Design review of the part built by this model. Coordinates are the model's own, in mm. Face numbers are marked on the shaded views. A direction names the side the tool comes from. Give positions to 0.01 mm unless a question says otherwise; leave off trailing zeros. Order: outer loops, then holes, each group sorted by start corner. A loop starts at its lowest first (then second) coordinate and runs counter-clockwise, first axis right, second up. Notation, with made-up numbers: (63.25, 89.25) - (97.25, 89.25) arc R21 cw to (97.25, 117.25) - close; hole circle Ø5 at (-13, 58.5). An arc over 180 degrees is marked (long way). Write each question's results on one line, items separated by ' | '. Start each with the question number.
```python
from build123d import *

# Parameters (mm, degrees)
F0_R     = 50
F0_R_2   = 15
F4_DEPTH = 30
F1_T     = -2.5
F2_W     = 3
F2_H     = 99.95499
F5_DEPTH = 27.5


with BuildPart() as f4:
    # F0 (on Top) → F4 (new body)
    with BuildSketch(Plane.XY):
        Circle(F0_R)
        Circle(F0_R_2, mode=Mode.SUBTRACT)
    extrude(amount=F4_DEPTH)

    # F1
    f1_openings = [f4.faces().sort_by_distance(p)[0] for p in [
        (-48.585786, 0, 30),
    ]]
    offset(amount=F1_T, openings=f1_openings)

    # F2 (on face) → F5 (join)
    with BuildSketch(Plane.XY.offset(2.5)):
        Rectangle(F2_W, F2_H)
    extrude(amount=F5_DEPTH)


solid = f4.part
```
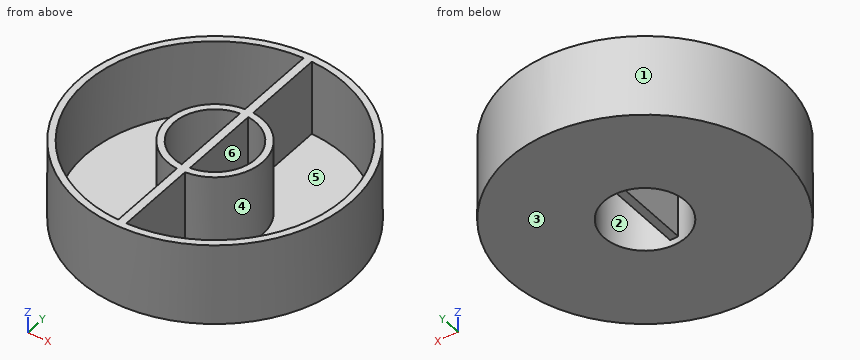
Q1. Add section B-B (y = 0). Give the boundary of the cut face in (x, z).
Q2. Add section C-C (x = 8). Give the boundary of the cut face in (y, z), plus the area to 3 significant figures.
Q3. Machinability: for the marked faces 5 and 6, which of the approach directions +Z, -Z, +X, -X, +Y, -Y give a long, thin tool a straight path to every point of the face, cutting with its end or side? Answer none if there is none.
Q4. Draft analysis for pull direction X (two halves, no side actions). For the marked faces 1, 2, 3 and 4, state which applies: pulls with the +X half, pulls with the -X half, needs draft (parallel to the pull), parting line crosses it, or undercut.
Q5. Insertion check: pin 1 Ø14 at (y, z) = (39.5, 16.5) entering from +X; pin 2 Ø2 at (x, z) = (22, 27) entering from -Y; pin 3 Ø4 at (x, y) = (-7, 31.5) entering from -Z; pin 4 Ø4 at (y, z) = (-24, 18.5) entering from +X. Each pin has a flat end and moves straight along its axis. Give the tip position at first contact, or say it passes through.
Q6. Add section D-D (y = -27). Give the boundary of the cut face in (x, z), plus the area to 3 significant figures.
Q7. For line 1 (X direction, y = 0, z = 6.75); line 2 (X direction, y = 26, z = 12.5); line 3 (X direction, y = 8, z = 19.25), list the stretches that pass through material, from the lowest coordinate up. Write a range as [from, to].
Verdict:
1) outline: (-50, 0) - (-15, 0) - (-15, 30) - (-17.5, 30) - (-17.5, 2.5) - (-47.5, 2.5) - (-47.5, 30) - (-50, 30) - close; (-1.5, 2.5) - (1.5, 2.5) - (1.5, 30) - (-1.5, 30) - close; (15, 0) - (50, 0) - (50, 30) - (47.5, 30) - (47.5, 2.5) - (17.5, 2.5) - (17.5, 30) - (15, 30) - close
2) outline: (-49.36, 0) - (-12.69, 0) - (-12.69, 30) - (-15.56, 30) - (-15.56, 2.5) - (-46.82, 2.5) - (-46.82, 30) - (-49.36, 30) - close; (12.69, 0) - (49.36, 0) - (49.36, 30) - (46.82, 30) - (46.82, 2.5) - (15.56, 2.5) - (15.56, 30) - (12.69, 30) - close | area: 481 mm2
3) face 5: +Z | face 6: +Z, -Z
4) face 1: parting line crosses it | face 2: undercut | face 3: needs draft | face 4: undercut
5) pin 1: stops at x = 38 | pin 2: stops at y = -45.38 | pin 3: stops at z = 0 | pin 4: stops at x = 44.9
6) outline: (-42.08, 0) - (42.08, 0) - (42.08, 30) - (39.08, 30) - (39.08, 2.5) - (1.5, 2.5) - (1.5, 30) - (-1.5, 30) - (-1.5, 2.5) - (-39.08, 2.5) - (-39.08, 30) - (-42.08, 30) - close | area: 458 mm2
7) line 1: x = [-50, -47.5], [-17.5, -15], [-1.5, 1.5], [15, 17.5], [47.5, 50] | line 2: x = [-42.71, -39.75], [-1.5, 1.5], [39.75, 42.71] | line 3: x = [-49.36, -46.82], [-15.56, -12.69], [-1.5, 1.5], [12.69, 15.56], [46.82, 49.36]
